```python
from build123d import *

# Parameters (mm, degrees)
F1_DEPTH = 6
F2_W     = 10
F2_H     = 12.1811708808
F2_R     = 4
F2_R_2   = 5
F2_R_3   = 2
F2_H_2   = 27.5950810313
F3_DEPTH = 25
F5_DEPTH = 3


with BuildPart() as f1:
    # F0 (on Top) → F1 (new body)
    with BuildSketch(Plane.XY):
        with BuildLine():
            Line((20, 110), (-20, 110))
            ThreePointArc((-20, 110), (-23.5355339059, 108.5355339059), (-25, 105))
            Line((-25, 105), (-25, -105))
            ThreePointArc((-25, -105), (-23.5355339059, -108.5355339059), (-20, -110))
            Line((-20, -110), (20, -110))
            ThreePointArc((20, -110), (23.5355339059, -108.5355339059), (25, -105))
            Line((25, -105), (25, 105))
            ThreePointArc((25, 105), (23.5355339059, 108.5355339059), (20, 110))
        make_face()
    extrude(amount=F1_DEPTH)

    # F2 (on face) → F3 (cut)
    with BuildSketch(Plane.XY.offset(6)):
        with Locations((0, -103.9094145596)):
            Rectangle(F2_W, F2_H)
        with BuildLine():
            Line((-5, -97.8188291192), (5, -97.8188291192))
            Line((5, -97.8188291192), (5, -70))
            ThreePointArc((5, -70), (0, -65), (-5, -70))
            Line((-5, -70), (-5, -97.8188291192))
        make_face()
        with Locations((0, -10)):
            Circle(F2_R)
        with Locations((0, 34.5)):
            Circle(F2_R_2)
        with Locations((-15, 50)):
            Circle(F2_R_3)
        with BuildLine():
            ThreePointArc((16.2007454783, 51.5994406198), (13, 50), (16.2007454783, 48.4005593802))
            Line((16.2007454783, 48.4005593802), (16.2007454783, 51.5994406198))
        make_face()
        with BuildLine():
            Line((5, 70), (5, 82.4049189687))
            Line((5, 82.4049189687), (-5, 82.4049189687))
            Line((-5, 82.4049189687), (-5, 70))
            ThreePointArc((-5, 70), (0, 65), (5, 70))
        make_face()
        with Locations((0, 96.2024594843)):
            Rectangle(F2_W, F2_H_2)
        with BuildLine():
            Line((16.2007454783, 51.5994406198), (16.2007454783, 48.4005593802))
            ThreePointArc((16.2007454783, 48.4005593802), (16.7890627374, 49.1059896412), (17, 50))
            ThreePointArc((17, 50), (16.7890627374, 50.8940103588), (16.2007454783, 51.5994406198))
        make_face()
    extrude(amount=-F3_DEPTH, mode=Mode.SUBTRACT)

    # F4 (on face) → F5 (cut)
    with BuildSketch(Plane.XY.offset(6)):
        Polygon((25, 60), (12.5, 60), (-25, 60), (-25, 40), (25, 40), align=None)
    extrude(amount=-F5_DEPTH, mode=Mode.SUBTRACT)


solid = f1.part
```
The listing builds one solid part. Answer for the finished solid, in the listing's coordinates (mm). A direction names the side the tool comes from. Coordinates: 2 decimals unless noted, no trailing zeros. Write each loop counter-clockwise with the first axis right and the second up, starting at its lowest first coordinate (ties: lowest second). Pieces come first, ordered by that corner, then holes. Notation, with made-up numbers: M 19,64 L 61,64 A5 cw 61,69 Z; hole C -2.75,6 d8. An arc over 180 degrees is marked long. Use a Markdown table: item, result. Add a question column.
1. Given P1, Ø6.5, axis at x = -15, y = 50, coming from the -Z side; P2, Ø3.5, axis at x = -1.5, z = 4, coming from the +Y side; P3, Ø16, axis at x = 5, y = 51, coming from the +Z side, each flat-ended and moving along its own axis, determine where each tip first touches the part or whether it passes through.
2. For a pull along X with two mould halves and no side action, classify faces 4 (the flat face through (-13, -110, 3)), 5 (the flat face through (-25, 1, 3)), 6 (the flat face through (-5, -90, 3)) as +X half, -X half, draft (parallel to the pull), parting line (faces both ways), or undercut.
3. Section D-D (x = 0) is taken. Give the vertices of the cut face in (y, z), plus the area to 3 significant figures.
4. Section B-B (y = -10) is taken. Give the vertices of the cut face in (x, z).
5. Which of the six approach directions +Z, -Z, +X, -X, +Y, -Y give full straight-line access (tool end or side, diameter ignored) to faces 1 (the flat face through (-5, 90, 3)), 2 (the flat face through (25, -1, 3)), 3 (the flat face through (5, -90, 3))?
6. Straight lines are drawn through the part: line 1 along Y through (x, z) = (0, 3.6); line 2 along X through (y, z) = (-85.5, 4.45); line 3 along Y through (x, z) = (20, 5.15). For each, find the intervals that lie inside material, in ascending order. Write a range as [from, to].
7. Section C-C (x = -15) is taken. Give the vertices of the cut face in (y, z), plus the area to 3 significant figures.
8. Section A-A (z = 4) is taken. Give the vertices of the cut face in (x, y), plus the area to 3 significant figures.
Data:
| question | item | result |
|---|---|---|
| 1 | P1 | stops at z = 0 |
| 1 | P2 | stops at y = 66.2 |
| 1 | P3 | stops at z = 3 |
| 2 | face 4 | draft |
| 2 | face 5 | -X half |
| 2 | face 6 | undercut |
| 3 | outline | M -65,0 L -14,0 L -14,6 L -65,6 Z; M -6,0 L 29.5,0 L 29.5,6 L -6,6 Z; M 39.5,0 L 65,0 L 65,6 L 60,6 L 60,3 L 40,3 L 40,6 L 39.5,6 Z |
| 3 | area | 612 mm2 |
| 4 | outline | M -25,0 L -4,0 L -4,6 L -25,6 Z; M 4,0 L 25,0 L 25,6 L 4,6 Z |
| 5 | face 1 | +Z, -Z, +Y |
| 5 | face 2 | +Z, -Z, +X, +Y, -Y |
| 5 | face 3 | +Z, -Z, -Y |
| 6 | line 1 | y = [-65, -14], [-6, 29.5], [39.5, 40], [60, 65] |
| 6 | line 2 | x = [-25, -5], [5, 25] |
| 6 | line 3 | y = [-110, 40], [60, 110] |
| 7 | outline | M -110,0 L 48,0 L 48,3 L 40,3 L 40,6 L -110,6 Z; M 52,0 L 110,0 L 110,6 L 60,6 L 60,3 L 52,3 Z |
| 7 | area | 1,250 mm2 |
| 8 | outline | M -25,-105 A5 ccw -20,-110 L -5,-110 L -5,-70 A5 cw 5,-70 L 5,-110 L 20,-110 A5 ccw 25,-105 L 25,40 L -25,40 Z; M -25,60 L 25,60 L 25,105 A5 ccw 20,110 L 5,110 L 5,70 A5 cw -5,70 L -5,110 L -20,110 A5 ccw -25,105 Z; hole C 0,34.5 d10; hole C 0,-10 d8 |
| 8 | area | 8,970 mm2 |
